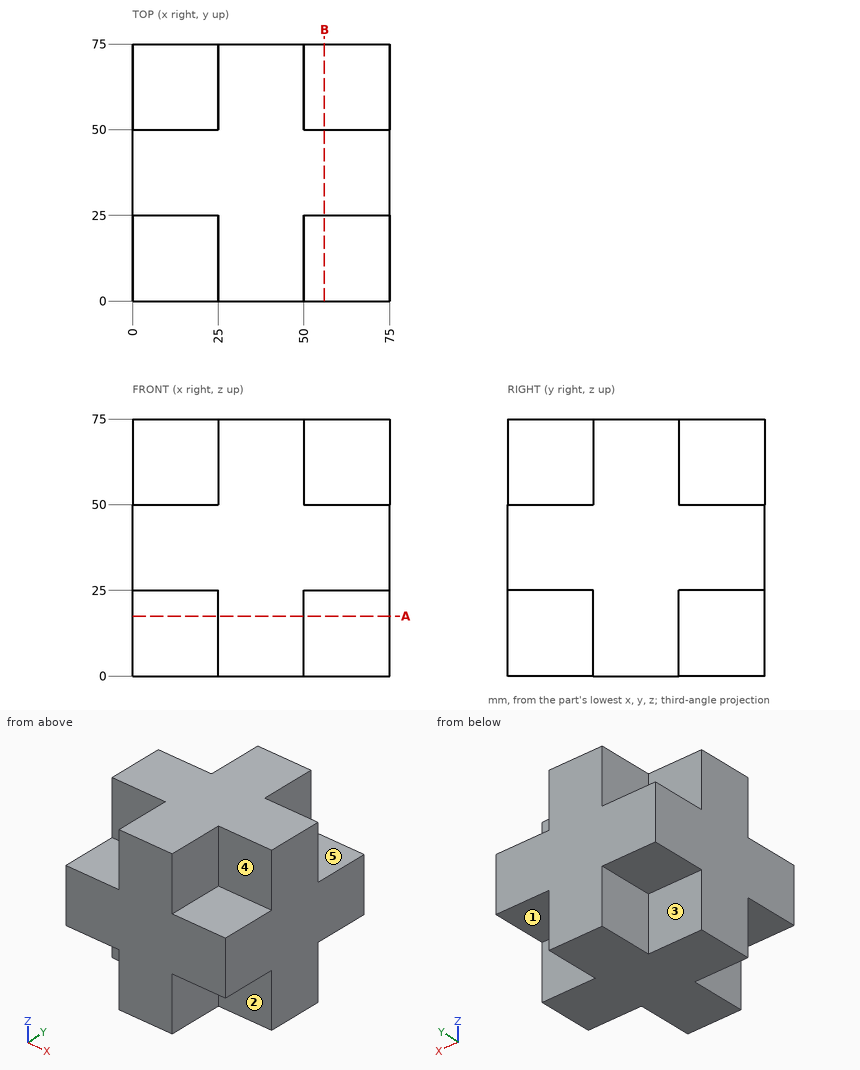
Check sheet for the drawn part. Datum: minimum x, y, z corner. Units: mm. A direction names the side the tool comes from. Give positions to 0.01 mm unless a question says otherwise; leave off trailing zeros. Order: outer loops, then holes, each group sorted by start corner. A loop starts at its lowest first (then second) coordinate and runs counter-clockwise, first axis right, second up. Notation, with made-up numbers: (37, -24.5) - (52, -24.5) arc R19 cw to (52, -4.5) - close; hole circle Ø6 at (-1.75, -4). An arc over 180 degrees is marked (long way). Answer in a Markdown table with one row per item. Add a question column.
Q1. Cross-section at A-A, the plane z = 17.5. Enter the section's corners in (x, y), then the cut area to 4 significant figures.
Q2. Tool access check on the marked faces 1, 2, 3, 4 and 5. Record the directions out of +Z, -Z, +X, -X, +Y, -Y that give a thin tool (end or side, any length) a straight path to the whole face; none if there is none.
Q3. Gauge pin test, flat ends, axial feed: pin 1 (7.5 mm diameter, centred on x = 7.5, z = 56.5, fed in from +Y); pin 2 (7.5 mm diameter, centred on x = 13, z = 7, fed in from -Y); pin 3 (12.5 mm diameter, centred on y = 11.5, z = 10, fed in from -X). Record the tip position at first contact, or that the pin passes through.
Q4. Material ranges on probe 1 along X at (y, z) = (60, 61), recorded low to high. Write a range as from..to.
Check values:
| question | item | result |
|---|---|---|
| 1 | outline | (0, 25) - (25, 25) - (25, 0) - (50, 0) - (50, 25) - (75, 25) - (75, 50) - (50, 50) - (50, 75) - (25, 75) - (25, 50) - (0, 50) - close |
| 1 | area | 3,125 mm^2 |
| 2 | face 1 | -Z, +X, +Y |
| 2 | face 2 | -Z, +X, -Y |
| 2 | face 3 | -Z, -X, +Y |
| 2 | face 4 | +Z, +X, -Y |
| 2 | face 5 | +Z, +X, +Y |
| 3 | pin 1 | stops at y = 50 |
| 3 | pin 2 | stops at y = 25 |
| 3 | pin 3 | stops at x = 25 |
| 4 | probe 1 | x = 25..50 |
